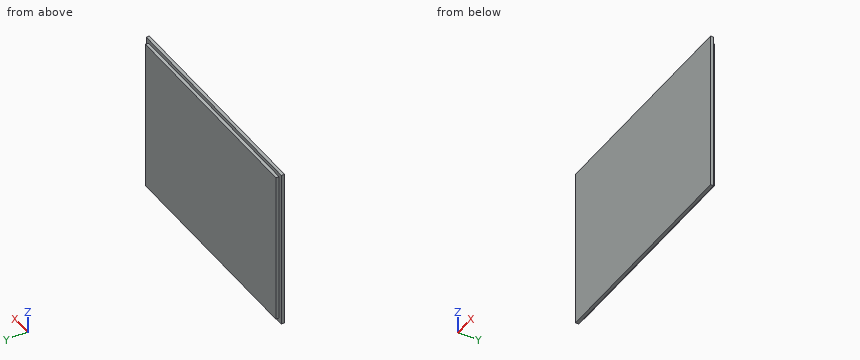
from build123d import *

# Parameters (mm, degrees)
CROQUIS1_W              = 72
CROQUIS1_H              = 52
CROQUIS1_W_2            = 69.5
CROQUIS1_H_2            = 49.5
SALIENTE_EXTRUIR1_DEPTH = 1
CROQUIS1_5_W            = 69.5
CROQUIS1_5_H            = 49.5
SALIENTE_EXTRUIR3_DEPTH = 2


with BuildPart() as part:
    # Croquis1 → Saliente-Extruir1 (new body)
    with BuildSketch(Plane(origin=(0, 0, 0), x_dir=(1, 0, 0), z_dir=(0, 1, 0))):
        with Locations((34.75, 24.75)):
            Rectangle(CROQUIS1_W, CROQUIS1_H)
        with Locations((34.75, 24.75)):
            Rectangle(CROQUIS1_W_2, CROQUIS1_H_2, mode=Mode.SUBTRACT)
    extrude(amount=SALIENTE_EXTRUIR1_DEPTH)

    # Croquis1<5> → Saliente-Extruir3 (add)
    with BuildSketch(Plane(origin=(0, 0, 0), x_dir=(1, 0, 0), z_dir=(0, 1, 0))):
        with Locations((34.75, 24.75)):
            Rectangle(CROQUIS1_5_W, CROQUIS1_5_H)
    extrude(amount=SALIENTE_EXTRUIR3_DEPTH)


solid = part.part
The listing builds one solid part. Answer for the finished solid, in the listing's coordinates (mm). Round coordinates to 2 decimals unless told otherwise and drop trailing zeros. Order: outer loops, then holes, each group sorted by start corner. A loop starts at its lowest first (then second) coordinate and runs counter-clockwise, first axis right, second up. Notation, with made-up numbers: (-17.5, -16) - (6.5, -16) arc R26 cw to (6.5, 4) - close; hole circle Ø9 at (-24, 6). An arc over 180 degrees is marked (long way). Write item = value, one per line. Start each with the question number.
1) Section A-A, the plane x = 22 is taken. Write down the section's boundary in (y, z), plus the area to 4 significant figures.
2) Straight lines are drawn through the part: L1, parallel to Z at x = 68, y = 1.45; L2, parallel to X at y = 1.35, z = -1. For each, find the intervals that lie inside material, in ascending order.
3) Given pin 1 (0.5 mm diameter, centred on x = 47, y = 1.5, fed in from +Z); pin 2 (0.8 mm diameter, centred on y = 1.5, z = -13.5, fed in from +X), each flat-ended and moving along its own axis, determine where each tip first touches the part or whether it passes through.
4) Section C-C, the plane y = 1.3 is taken. Write down the section's boundary in (x, z).
5) Section B-B, the plane z = -29 is taken. Write down the section's boundary in (x, y).
Results list:
q1.outline = (0, -50.75) - (1, -50.75) - (1, -49.5) - (2, -49.5) - (2, 0) - (1, 0) - (1, 1.25) - (0, 1.25) - close
q1.area = 101.5 mm^2
q2.L1 = -49.5 to 0
q2.L2 = 0 to 69.5
q3.pin_1 = 0
q3.pin_2 = 69.5
q4.outline = (0, -49.5) - (69.5, -49.5) - (69.5, 0) - (0, 0) - close
q5.outline = (-1.25, 0) - (70.75, 0) - (70.75, 1) - (69.5, 1) - (69.5, 2) - (0, 2) - (0, 1) - (-1.25, 1) - close
